```python
from build123d import *

# Parameters (mm, degrees)
F0_R     = 63.5
F1_DEPTH = 101.6
F2_SIZE  = 5.08
F4_DEPTH = 88.9
F6_DEPTH = 76.2
F8_DEPTH = 63.5
F9_DEPTH = 203.2
F11_R    = 7.62


with BuildPart() as f1:
    # F0 (on Top) → F1 (new body, symmetric)
    with BuildSketch(Plane.XY):
        Circle(F0_R)
    extrude(amount=F1_DEPTH, both=True)

    # F2
    f2_edges = [f1.edges().sort_by_distance(p)[0] for p in [
        (-63.5, 0, 101.6),
    ]]
    chamfer(f2_edges, length=F2_SIZE)

    # F3 (on Front) → F4 (join)
    with BuildSketch(Plane.XZ):
        with BuildLine():
            ThreePointArc((-27.294820104, 63.1642854473), (-36.184820104, 72.0542854473), (-45.074820104, 63.1642854473))
            Line((-45.074820104, 63.1642854473), (-45.074820104, 42.8442854473))
            ThreePointArc((-45.074820104, 42.8442854473), (-36.184820104, 33.9542854473), (-27.294820104, 42.8442854473))
            Line((-27.294820104, 42.8442854473), (-27.294820104, 63.1642854473))
        make_face()
        with BuildLine():
            ThreePointArc((45.070431488, 63.1642854473), (36.182625796, 72.0520911393), (27.294820104, 63.1642854473))
            Line((27.294820104, 63.1642854473), (27.294820104, 42.8442854473))
            ThreePointArc((27.294820104, 42.8442854473), (36.182625796, 33.9564797553), (45.070431488, 42.8442854473))
            Line((45.070431488, 42.8442854473), (45.070431488, 63.1642854473))
        make_face()
    extrude(amount=F4_DEPTH)

    # F5 (on Front) → F6 (join)
    with BuildSketch(Plane.XZ):
        with BuildLine():
            ThreePointArc((10.1674738791, 14.9895709281), (1.2774738791, 23.8795709281), (-7.6125261209, 14.9895709281))
            Line((-7.6125261209, 14.9895709281), (-7.6125261209, -10.4104290719))
            ThreePointArc((-7.6125261209, -10.4104290719), (1.2774738791, -19.3004290719), (10.1674738791, -10.4104290719))
            Line((10.1674738791, -10.4104290719), (10.1674738791, 14.9895709281))
        make_face()
    extrude(amount=F6_DEPTH)

    # F7 (on Front) → F8 (join)
    with BuildSketch(Plane.XZ):
        with BuildLine():
            Line((24.3475708148, -43.7428626594), (-21.3724291852, -43.7428626594))
            ThreePointArc((-21.3724291852, -43.7428626594), (-28.9924291852, -51.3628626594), (-21.3724291852, -58.9828626594))
            Line((-21.3724291852, -58.9828626594), (24.3475708148, -58.9828626594))
            ThreePointArc((24.3475708148, -58.9828626594), (31.9675708148, -51.3628626594), (24.3475708148, -43.7428626594))
        make_face()
    extrude(amount=F8_DEPTH)

    # F9 (cut, through all): a face of the model
    f9_faces = [f1.faces().sort_by_distance(p)[0] for p in [
        (0, 0, 101.6),
    ]]
    extrude(f9_faces, amount=-F9_DEPTH, mode=Mode.SUBTRACT)

    # F11
    f11_edges = [f1.edges().sort_by_distance(p)[0] for p in [
        (-36.18482, -88.9, 72.054285),
        (-27.29482, -88.9, 53.004285),
        (36.182626, -88.9, 33.95648),
        (27.29482, -88.9, 53.004285),
    ]]
    fillet(f11_edges, radius=F11_R)


solid = f1.part
```
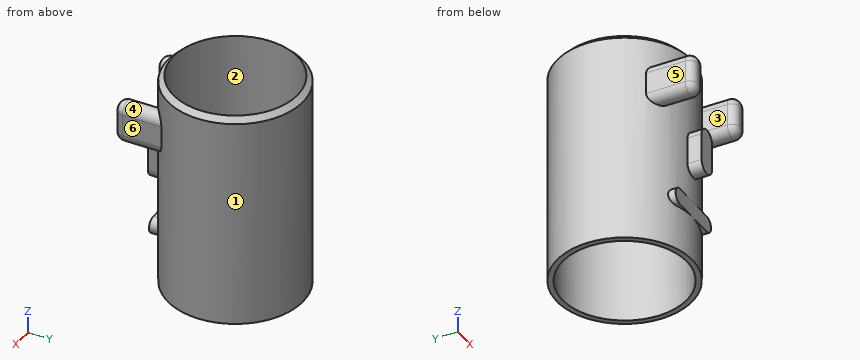
The model under review builds one solid part; all positions refer to its coordinate system, in mm. Face numbers are marked on the shaded views. A direction names the side the tool comes from. Round coordinates to 2 decimals unless told otherwise and drop trailing zeros. Order: outer loops, then holes, each group sorted by start corner. A loop starts at its lowest first (then second) coordinate and runs counter-clockwise, first axis right, second up.
(1) Tool access review of the marked faces 4, 5 and 6: name each direction out of +Z, -Z, +X, -X, +Y, -Y from which nothing blocks a thin tool from reaching the whole face with its end or side.
Working result:
face 4: +Z, -Y
face 5: +Z, -Z, -X, -Y
face 6: +Z, -Z, +X, -Y
(2) Wall thickness on L1, parallel to Y at x = 0, z = 6.5; L2, parallel to Y at x = 0, z = 44.5; L3, parallel to X at y = 3, z = 25.5: over which ranges is each line inside the solid? List them lowest first.
Working result:
L1: y = -76.2 to -58.42, 58.42 to 63.5
L2: y = -63.5 to -58.42, 58.42 to 63.5
L3: x = -63.43 to -58.34, 58.34 to 63.43
(3) Take a section at B-B, the plane z = 0. State the section outline as (x, y) points.
Working result:
outline: (-7.61, -76.2) - (10.17, -76.2) - (10.17, -62.68) arc R63.5 ccw (long way) to (-7.61, -63.04) - close; hole circle Ø116.84 at (0, 0)
(4) For P1, Ø12, axis at x = 46, z = 20, coming from the +Y side; P2, Ø6, axis at y = -64, z = 49, coming from the +X side; P3, Ø2.5, axis at x = 17, y = -61, coming from the +Z side, all flat-tipped, find the tip position at first contact; note any pin that passes through.
Working result:
P1: stops at y = 49.32
P2: stops at x = 45.07
P3: stops at z = 97.95
(5) Mouldability with a two-part tool opening along Y and no side actions: class the marked faces 1, 2 and 3 as released by +Y, released by -Y, zero draft, split by the parting line, or undercut.
Working result:
face 1: split by the parting line
face 2: undercut
face 3: zero draft
(6) Take a section at C-C, the plane z = -51. State the section outline as (x, y) points.
Working result:
outline: (-28.98, -63.5) - (31.96, -63.5) - (31.96, -54.87) arc R63.5 ccw (long way) to (-28.98, -56.5) - close; hole circle Ø116.84 at (0, 0)
(7) Take a section at A-A, the plane y = 0. State the section outline as (x, z) points, plus the area to 3 significant figures.
Working result:
outline: (-63.5, -101.6) - (-58.42, -101.6) - (-58.42, 101.6) - (-63.5, 96.52) - close; (58.42, -101.6) - (63.5, -101.6) - (63.5, 96.52) - (58.42, 101.6) - close
area: 2,040 mm2
